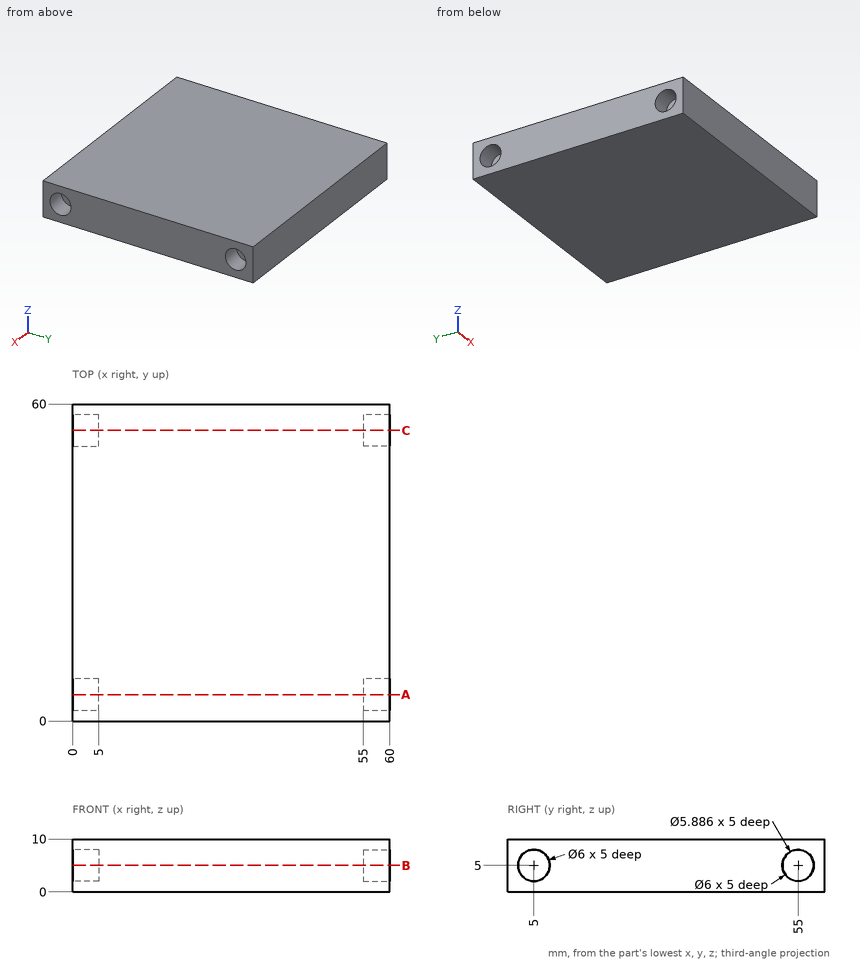
Can you work these out from the drawing? Everything is in mm from the part's minimum corner. Give positions to 0.01 mm unless a question says otherwise; leave off trailing zeros. Write each loop counter-clockwise with the first axis right and the second up, starting at its lowest first coordinate (ties: lowest second). Pieces come first, ordered by that corner, then holes. Notation, with made-up numbers: (16.25, 47.25) -> (22.25, 47.25) arc R25 ccw to (22.25, 84.25) -> close; hole circle Ø8 at (-10.5, 33.25). An arc over 180 degrees is marked (long way). Write each question's results on one line, items separated by ' | '. Start each with the question number.
Q1. Suppose I cut it at C-C, the plane y = 55. List the corners of the cut face in (x, z) for me.
Q2. I'm going to push flat-ended pins straight in: pin 1 Ø3.5 at (y, z) = (5, 5) entering from +X; pin 2 Ø5 at (y, z) = (55, 5) entering from -X. Where does each tip first touch, or does it pass through?
Q3. Suppose I cut it at A-A, the plane y = 5. List the corners of the cut face in (x, z) for me.
Q4. Suppose I cut it at B-B, the plane z = 5. List the corners of the cut face in (x, y) for me.
Q5. I need wall thicknesses on probe 1 along Z at (x, y) = (58.55, 5); probe 2 along Y at (x, z) = (3, 7.75) (1 decimal); probe 3 along Y at (x, z) = (57.5, 7) (1 decimal). Which ranges of each line are inside material? Lowest first, please.
Outcome:
1) outline: (0, 0) -> (60, 0) -> (60, 2.06) -> (55, 2.06) -> (55, 7.94) -> (60, 7.94) -> (60, 10) -> (0, 10) -> (0, 8) -> (5, 8) -> (5, 2) -> (0, 2) -> close
2) pin 1: x = 55 | pin 2: x = 5
3) outline: (0, 0) -> (60, 0) -> (60, 2) -> (55, 2) -> (55, 8) -> (60, 8) -> (60, 10) -> (0, 10) -> (0, 8) -> (5, 8) -> (5, 2) -> (0, 2) -> close
4) outline: (0, 0) -> (60, 0) -> (60, 2) -> (55, 2) -> (55, 8) -> (60, 8) -> (60, 52.06) -> (55, 52.06) -> (55, 57.94) -> (60, 57.94) -> (60, 60) -> (0, 60) -> (0, 58) -> (5, 58) -> (5, 52) -> (0, 52) -> (0, 8) -> (5, 8) -> (5, 2) -> (0, 2) -> close
5) probe 1: 0 to 2, 8 to 10 | probe 2: 0 to 3.8, 6.2 to 53.8, 56.2 to 60 | probe 3: 0 to 2.8, 7.2 to 52.8, 57.2 to 60
